Verification items for the finished model (mm, model axes). Coordinates: 2 decimals unless noted, no trailing zeros. Order: outer loops, then holes, each group sorted by start corner. A loop starts at its lowest first (then second) coordinate and runs counter-clockwise, first axis right, second up. Notation, with made-up numbers: (19.25, 19.5) -> (57.25, 19.5) arc R16 ccw to (57.25, 48.5) -> close; hole circle Ø5 at (-25.5, 50). An arc over 180 degrees is marked (long way). Answer as CSV lines item,"result".
Autodesk Inventor part; units mm, degrees
ref_plane "YZ Plane" through (0, 0, 0) normal (1, 0, 0) x (0, 1, 0)
ref_plane "XZ Plane" through (0, 0, 0) normal (0, 1, 0) x (-1, 0, 0)
sketch "Sketch1" plane through (0, 0, 0) normal (1, 0, 0) x (0, 1, 0)
  circle A0 centre (0, -124) radius 1.95
  circle A1 centre (0, 124) radius 1.95
  circle A2 centre (-19, -65) radius 1.5
  circle A3 centre (-19, 65) radius 1.5
  line L0 (0, 124) -> (-19, 65) construction
  line L1 (4.7593, 122.4673) -> (-14.2407, 63.4673)
  line L2 (-23.7593, 66.5327) -> (-4.7593, 125.5327)
  arc A4 (4.7593, 122.4673) -> (-4.7593, 125.5327) centre (0, 124) ccw
  arc A5 (-23.7593, 66.5327) -> (-14.2407, 63.4673) centre (-19, 65) ccw
  line L3 (-19, 65) -> (-19, -65) construction
  line L4 (-24, 65) -> (-24, -65)
  line L5 (-14, -65) -> (-14, 65)
  arc A6 (-14, 65) -> (-24, 65) centre (-19, 65) ccw
  arc A7 (-24, -65) -> (-14, -65) centre (-19, -65) ccw
  line L6 (-19, -65) -> (0, -124) construction
  line L7 (-23.7593, -66.5327) -> (-4.7593, -125.5327)
  line L8 (4.7593, -122.4673) -> (-14.2407, -63.4673)
  arc A8 (-14.2407, -63.4673) -> (-23.7593, -66.5327) centre (-19, -65) ccw
  arc A9 (-4.7593, -125.5327) -> (4.7593, -122.4673) centre (0, -124) ccw
  circle A10 centre (-44, 65) radius 1.5
  circle A11 centre (-44, -65) radius 1.5
  line L9 (-19, 65) -> (-44, 65) construction
  line L10 (-19, 70) -> (-44, 70)
  line L11 (-44, 60) -> (-19, 60)
  arc A12 (-19, 60) -> (-19, 70) centre (-19, 65) ccw
  arc A13 (-44, 70) -> (-44, 60) centre (-44, 65) ccw
  line L12 (-19, -65) -> (-44, -65) construction
  line L13 (-19, -60) -> (-44, -60)
  line L14 (-44, -70) -> (-19, -70)
  arc A14 (-19, -70) -> (-19, -60) centre (-19, -65) ccw
  arc A15 (-44, -60) -> (-44, -70) centre (-44, -65) ccw
  line L15 (0, 124) -> (-44, 65) construction
  line L16 (-4.0081, 126.9891) -> (-48.0081, 67.9891)
  line L17 (-39.9919, 62.0109) -> (4.0081, 121.0109)
  arc A16 (4.0081, 121.0109) -> (-4.0081, 126.9891) centre (0, 124) ccw
  arc A17 (-48.0081, 67.9891) -> (-39.9919, 62.0109) centre (-44, 65) ccw
  line L18 (-44, -65) -> (0, -124) construction
  line L19 (-48.0081, -67.9891) -> (-4.0081, -126.9891)
  line L20 (4.0081, -121.0109) -> (-39.9919, -62.0109)
  arc A18 (-39.9919, -62.0109) -> (-48.0081, -67.9891) centre (-44, -65) ccw
  arc A19 (-4.0081, -126.9891) -> (4.0081, -121.0109) centre (0, -124) ccw
  line L21 (-44, 65) -> (-44, -65) construction
  line L22 (-49, 65) -> (-49, -65)
  line L23 (-39, -65) -> (-39, 65)
  arc A20 (-39, 65) -> (-49, 65) centre (-44, 65) ccw
  arc A21 (-49, -65) -> (-39, -65) centre (-44, -65) ccw
  line L24 (-44, 65) -> (-19, 0) construction
  line L25 (-45.4, 64.4615) -> (-20.4, -0.5385)
  line L26 (-17.6, 0.5385) -> (-42.6, 65.5385)
  arc A22 (-42.6, 65.5385) -> (-45.4, 64.4615) centre (-44, 65) ccw
  arc A23 (-20.4, -0.5385) -> (-17.6, 0.5385) centre (-19, 0) ccw
  line L27 (-44, -65) -> (-19, 0) construction
  line L28 (-42.6, -65.5385) -> (-17.6, -0.5385)
  line L29 (-20.4, 0.5385) -> (-45.4, -64.4615)
  arc A24 (-45.4, -64.4615) -> (-42.6, -65.5385) centre (-44, -65) ccw
  arc A25 (-17.6, -0.5385) -> (-20.4, 0.5385) centre (-19, 0) ccw
  line L30 (-19, 0) -> (-44, 0) construction
  line L31 (-19, 1.5) -> (-44, 1.5)
  line L32 (-44, -1.5) -> (-19, -1.5)
  arc A26 (-19, -1.5) -> (-19, 1.5) centre (-19, 0) ccw
  arc A27 (-44, 1.5) -> (-44, -1.5) centre (-44, 0) ccw
  circle A28 centre (-19, -10) radius 1.5
  circle A29 centre (-19, -35) radius 1.5
  circle A30 centre (-19, 10) radius 1.5
  circle A31 centre (-19, 35) radius 1.5
  point P0 (0, 0)
  point P1 (-9.5, 94.5)
  point P2 (-9.5, -94.5)
  point P3 (-14, -64.2148)
  point P4 (-14, 64.2148)
  point P5 (-24, 65)
  point P6 (-31.5, 65)
  point P7 (-31.5, -65)
  point P8 (-22, 94.5)
  point P9 (-22, -94.5)
  point P10 (-44, 0)
  point P11 (-31.5, 32.5)
  point P12 (-31.5, -32.5)
  point P13 (-39, 47.8215)
  point P14 (-24, 8.8215)
  point P15 (-24, 17.1785)
  point P16 (-40.4698, 60)
  point P17 (-24, 60)
  point P18 (-22.6427, 70)
  point P19 (-34.0339, 70)
  point P20 (-13.9854, 96.8832)
  point P21 (-6.8749, 118.9633)
  point P22 (-43.3898, 70)
  point P23 (-49, 65)
  point P24 (-43.3898, -70)
  point P25 (-6.8749, -118.9633)
  point P26 (-13.9854, -96.8832)
  point P27 (-34.0339, -70)
  point P28 (-22.6427, -70)
  point P29 (-24, -60)
  point P30 (-40.4698, -60)
  point P31 (-24, -17.1785)
  point P32 (-24, -8.8215)
  point P33 (-39, -47.8215)
  point P34 (-31.5, 0)
  point P35 (-39, -1.5)
  point P36 (-24, -1.5)
  point P37 (-24, 1.5)
  point P38 (-39, 1.5)
  point P39 (-49, 65)
  point P40 (-4.0081, -126.9891)
  point P41 (-39, 60)
  point P42 (-39, -60)
  point P43 (-39, -56.1785)
  point P44 (-39, 56.1785)
  dimension "d2" = 3.9
  dimension "d4" = 3.9
  dimension "d25" = 3
  dimension "d28" = 3
  dimension "d43" = 59
  dimension "d44" = 65
  dimension "d45" = 65
  dimension "d47" = 59
  dimension "d48" = 10
  dimension "d49" = 10
  dimension "d50" = 10
  dimension "d52" = 14
  dimension "d53" = 3
  dimension "d54" = 3
  dimension "d55" = 10
  dimension "d56" = 10
  dimension "d57" = 25
  dimension "d58" = 25
  dimension "d59" = 10
  dimension "d60" = 10
  dimension "d61" = 10
  dimension "d62" = 3
  dimension "d63" = 3
  dimension "d64" = 3
  dimension "d65" = 3
  dimension "d66" = 3
  dimension "d67" = 10
  dimension "d68" = 25
  dimension "d69" = 3
  dimension "d70" = 3
  dimension "d71" = 10
  dimension "d72" = 25
extrude "Extrusion1" add sketch "Sketch1" along normal blind 5 contours A16 L17 L2 A4 | L1 L5 A6 L10 L2 L17 A16 | L5 L8 A8 L13 L4 L28 A23 L26 L11 A5 L1 | L1 A12 L5 | A4 L2 L17 L10 A13 L16 | A5 A6 A12 | L8 A19 L20 L7 L14 A7 L5 | L5 A14 L8 | A13 A20 L23 L17 A17 L26 A10 L25 | L11 L4 A5 | A7 A8 A14 | A9 L7 L20 A19 | A6 L2 L10 | L10 L17 L23 A20 | A13 L11 L25 L23 L31 A27 L32 L29 L13 A15 L22 | L2 A5 L4 L11 L23 L17 L10 | L14 L7 A7 | L19 A15 L14 L20 L7 A9 | A8 L4 L13 | A17 L25 L11 | A15 A18 L29 A11 L28 L20 L23 A21 | L23 L11 L26 A17 L17 | L26 A25 L31 L25 L4 | L4 L25 L23 L26 | L23 L26 L11 | L7 L14 L20 L23 L13 L4 A7 | L25 A17 L26 L11 | L11 L26 L23 L25 | L25 A10 L26 A17 | L13 L29 A18 | L25 L31 L4 | A23 L25 L29 A25 | L14 A21 L23 L20 | L28 L23 L29 L4 | L4 L29 L32 A23 L28 | L23 L20 A18 L28 L13 | L13 L28 L23 | L29 L23 L28 L13 | L13 L28 A18 L29 | A18 L28 A11 L29 | L31 L25 L29 L32 L4 | L4 L32 L23 L31 | L31 A25 L29 L25 | L4 L32 L29 | L23 L32 A27 L31 | L25 A23 L32 L29
sketch "Sketch7" plane through (5, 0, 0) normal (1, 0, 0) x (0, 0, -1)
  circle A0 centre (-65, -19) radius 1.5
  circle A1 centre (-35, -19) radius 1.5
  circle A2 centre (-10, -19) radius 1.5
  circle A3 centre (35, -19) radius 1.5
  circle A4 centre (10, -19) radius 1.5
  circle A5 centre (65, -19) radius 1.5
  circle A6 centre (124, 0) radius 1.95
  line L0 (-17.1785, -24) -> (-56.1785, -39)
  line L1 (-56.1785, -39) -> (-60, -39)
  line L2 (-60, -39) -> (-60, -24)
  line L3 (-60, -24) -> (-17.1785, -24)
  circle A7 centre (65, -44) radius 1.5
  circle A8 centre (-65, -44) radius 1.5
  line L4 (-96.8832, -13.9854) -> (-70, -22.6427)
  line L5 (-70, -22.6427) -> (-70, -34.0339)
  line L6 (-70, -34.0339) -> (-96.8832, -13.9854)
  line L7 (-1.5, -39) -> (-47.8215, -39)
  line L8 (-47.8215, -39) -> (-8.8215, -24)
  line L9 (-8.8215, -24) -> (-1.5, -24)
  line L10 (-1.5, -24) -> (-1.5, -39)
  line L11 (8.8215, -24) -> (47.8215, -39)
  line L12 (47.8215, -39) -> (1.5, -39)
  line L13 (1.5, -39) -> (1.5, -24)
  line L14 (1.5, -24) -> (8.8215, -24)
  line L15 (60, -24) -> (60, -39)
  line L16 (60, -39) -> (56.1785, -39)
  line L17 (56.1785, -39) -> (17.1785, -24)
  line L18 (17.1785, -24) -> (60, -24)
  line L19 (96.8832, -13.9854) -> (70, -34.0339)
  line L20 (70, -34.0339) -> (70, -22.6427)
  line L21 (70, -22.6427) -> (96.8832, -13.9854)
  arc A9 (126.9891, -4.0081) -> (122.4673, 4.7593) centre (124, 0) ccw
  line L22 (122.4673, 4.7593) -> (64.2148, -14)
  line L23 (64.2148, -14) -> (-64.2148, -14)
  line L24 (-64.2148, -14) -> (-122.4673, 4.7593)
  arc A10 (-122.4673, 4.7593) -> (-126.9891, -4.0081) centre (-124, 0) ccw
  line L25 (-126.9891, -4.0081) -> (-67.9891, -48.0081)
  arc A11 (-67.9891, -48.0081) -> (-65, -49) centre (-65, -44) ccw
  line L26 (-65, -49) -> (65, -49)
  arc A12 (65, -49) -> (67.9891, -48.0081) centre (65, -44) ccw
  line L27 (67.9891, -48.0081) -> (126.9891, -4.0081)
  circle A13 centre (-124, 0) radius 1.95
  point P0 (0, 0)
properties part number "Horizontal_bar_V2"
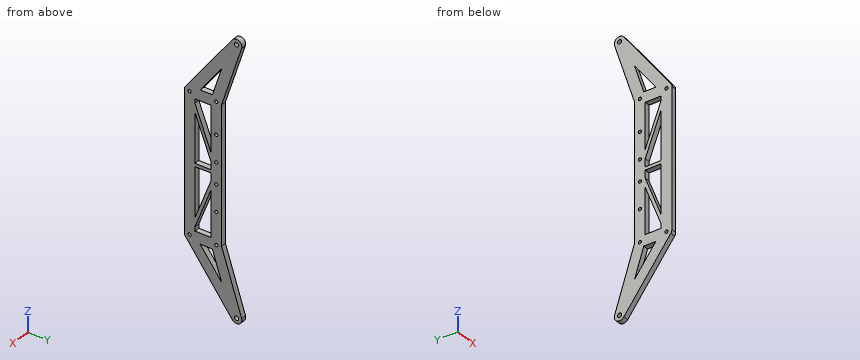
Item 1: Thickness scan on line 1 (Z direction, x = 3.15, y = -43); line 2 (Y direction, x = 3.95, z = 22); line 3 (Y direction, x = 1, z = 65). Record the ranges inside material, lowest first.
Answer list:
line 1,"-74.7 to -66.12, -63.88 to 63.88, 66.12 to 74.7"
line 2,"-49 to -39, -29.07 to -25.85, -24 to -14"
line 3,"-49 to -45.5, -42.5 to -20.5, -17.5 to -13.75"
Item 2: Section check A-A, the plane y = -10. Record the boundary of the cut face in (x, z), plus the area to 3 significant figures.
Answer list:
outline,"(0, -118.95) -> (5, -118.95) -> (5, -76.64) -> (0, -76.64) -> close; (0, 76.64) -> (5, 76.64) -> (5, 118.95) -> (0, 118.95) -> close"
area,"423 mm2"
Item 3: Section check B-B, the plane z = 40. Record the boundary of the cut face in (x, y).
Answer list:
outline,"(0, -49) -> (5, -49) -> (5, -39) -> (0, -39) -> close; (0, -35.99) -> (5, -35.99) -> (5, -32.78) -> (0, -32.78) -> close; (0, -24) -> (5, -24) -> (5, -14) -> (0, -14) -> close"
Item 4: Depth check by flat-ended pin: pin 1 Ø3 at (x, z) = (1.5, 58) entering from +Y; pin 2 Ø1 at (x, y) = (3.5, -32.5) entering from +Z; pin 3 Ø1 at (y, z) = (-37, 54) entering from -X; pin 4 Ø1 at (x, y) = (2, -33) entering from -Z. Enter the tip coordinate at first touch or a pass-through.
Answer list:
pin 1,"y = -14"
pin 2,"z = 89.45"
pin 3,"through"
pin 4,"z = -88.78"
Item 5: Section check C-C, the plane z = 80.5. Record the boundary of the cut face in (x, y).
Answer list:
outline,"(0, -38.68) -> (5, -38.68) -> (5, -26.2) -> (0, -26.2) -> close; (0, -19.26) -> (5, -19.26) -> (5, -8.76) -> (0, -8.76) -> close"
Item 6: Section check D-D, the plane y = -26.5. Record the boundary of the cut face in (x, z).
Answer list:
outline,"(0, -96.83) -> (5, -96.83) -> (5, -80.1) -> (0, -80.1) -> close; (0, -70) -> (5, -70) -> (5, -60) -> (0, -60) -> close; (0, -23.68) -> (5, -23.68) -> (5, -15.32) -> (0, -15.32) -> close; (0, -1.5) -> (5, -1.5) -> (5, 1.5) -> (0, 1.5) -> close; (0, 15.32) -> (5, 15.32) -> (5, 23.68) -> (0, 23.68) -> close; (0, 60) -> (5, 60) -> (5, 70) -> (0, 70) -> close; (0, 80.1) -> (5, 80.1) -> (5, 96.83) -> (0, 96.83) -> close"
